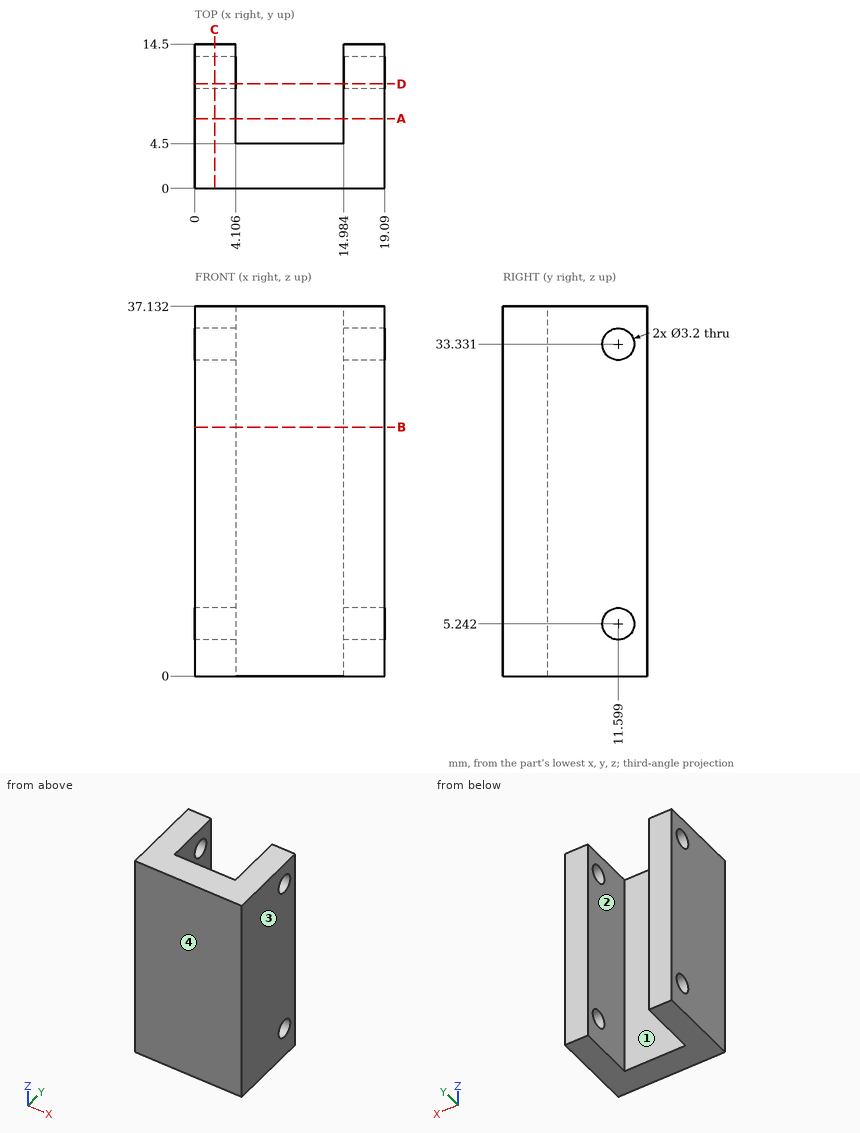
Source: three-view drawing plus pictorial views. Frame: mm from the lowest corner of the part. Give positions to 0.01 mm unless a question says otherwise; leave off trailing zeros. Loops run counter-clockwise (first coordinate to the right, second up) from the corner with the lowest first, then second, coordinate; pieces in that order, holes last.
1) Mould query, pull axis X, two halves, no side actions, for the marked faces 1, 2, 3 and 4. Classes: released by +X, released by -X, zero draft, split by the parting line, or undercut.
A:
face 1: undercut
face 2: undercut
face 3: released by +X
face 4: zero draft
2) Section query B-B on z = 25. Return the cut outline in (x, y), and give its area (3 significant figures).
A:
outline: (0, 0) - (19.09, 0) - (19.09, 14.5) - (14.98, 14.5) - (14.98, 4.5) - (4.11, 4.5) - (4.11, 14.5) - (0, 14.5) - close
area: 168 mm2
3) Section query D-D on y = 10.5. Return the cut outline in (x, z) (1 decimal), and give its area (3 significant figures).
A:
outline: (0, 0) - (4.1, 0) - (4.1, 4.1) - (0, 4.1) - close; (0, 6.4) - (4.1, 6.4) - (4.1, 32.2) - (0, 32.2) - close; (0, 34.5) - (4.1, 34.5) - (4.1, 37.1) - (0, 37.1) - close; (15, 0) - (19.1, 0) - (19.1, 4.1) - (15, 4.1) - close; (15, 6.4) - (19.1, 6.4) - (19.1, 32.2) - (15, 32.2) - close; (15, 34.5) - (19.1, 34.5) - (19.1, 37.1) - (15, 37.1) - close
area: 267 mm2
4) Contact query for flat-ended pins moving along their axis: pin 1 (5 mm diameter, centred on y = 11, z = 11.5, fed in from -X); pin 2 (6 mm diameter, centred on x = 9, z = 16, fed in from +Y). Output: stop coordinate, or through.
A:
pin 1: stops at x = 0
pin 2: stops at y = 4.5
5) Line query: L1, parallel to X at y = 7.5, z = 2; L2, parallel to Z at x = 4, y = 12.5 (1 decimal); L3, parallel to Y at x = 14, z = 13.5. Output: solid intervals per line, ascending.
A:
L1: x = 0 to 4.11, 14.98 to 19.09
L2: z = 0 to 3.9, 6.6 to 32, 34.7 to 37.1
L3: y = 0 to 4.5
6) Section query A-A on y = 7. Return the cut outline in (x, z).
A:
outline: (0, 0) - (4.11, 0) - (4.11, 37.13) - (0, 37.13) - close; (14.98, 0) - (19.09, 0) - (19.09, 37.13) - (14.98, 37.13) - close
7) Section query C-C on x = 2. Return the cut outline in (y, z), and give its area (3 significant figures).
A:
outline: (0, 0) - (14.5, 0) - (14.5, 37.13) - (0, 37.13) - close; hole circle Ø3.2 at (11.6, 5.24); hole circle Ø3.2 at (11.6, 33.33)
area: 522 mm2
